The listing builds one solid part. Answer for the finished solid, in the listing's coordinates (mm). Round coordinates to 2 decimals unless told otherwise and drop trailing zeros. Loops run counter-clockwise (first coordinate to the right, second up) from the corner with the lowest first, then second, coordinate; pieces in that order, holes last. Notation, with made-up numbers: (60.5, -39.75) -> (86.5, -39.75) arc R14 ccw to (86.5, -17.75) -> close; hole circle Ø6 at (6.25, 65). An arc over 180 degrees is marked (long way). Use a Markdown table: item, result. Add a question column.
Q1. Section D-D on x = -4.75 is taken. Give the vertices of the cut face in (y, z).
Q2. Consider line 1 (X direction, y = 5.75, z = 0); line 2 (Z direction, x = -2.25, y = -1). Determine where each line is inside the solid, lowest interval first.
Q3. Section C-C on y = -1.5 is taken. Give the vertices of the cut face in (x, z), then the cut area to 3 significant figures.
Q4. Given pin 1 Ø8 at (y, z) = (-4.5, -6) entering from -X; pin 2 Ø5 at (x, y) = (3.5, -5) entering from -Z; pin 3 Ø5 at (y, z) = (4.5, -4) entering from -X, each flat-ended and moving along its own axis, determine where each tip first touches the part or whether it passes through.
Q5. Section A-A on x = 0 is taken. Give the vertices of the cut face in (y, z), then the cut area to 3 significant figures.
Q6. Section B-B on z = 1 is taken. Give the vertices of the cut face in (x, y).
from build123d import *

# Parameters (mm, degrees)
ESBO_O1_R                = 9.5
ESBO_O1_R_2              = 3.25
ESBO_O1_R_3              = 2.75
RESSALTO_EXTRUS_O1_DEPTH = 11


with BuildPart() as part:
    # Esboço1 → Ressalto-extrusão1 (new, symmetric)
    # profile 1 of 2: a face of its own
    with BuildSketch(Plane(origin=(0, 0, 0), x_dir=(1, 0, 0), z_dir=(0, 1, 0))):
        with Locations(Location((0, 0, 0), (0, 0, 270))):
            Circle(ESBO_O1_R)
        Circle(ESBO_O1_R_2, mode=Mode.SUBTRACT)
    # profile 2 of 2: a face of its own
    with BuildSketch(Plane(origin=(0, 0, 0), x_dir=(1, 0, 0), z_dir=(0, 1, 0))):
        Circle(ESBO_O1_R_2)
        with Locations(Location((0, 0, 0), (0, 0, 270))):
            Circle(ESBO_O1_R_3, mode=Mode.SUBTRACT)
    extrude(amount=RESSALTO_EXTRUS_O1_DEPTH, both=True)


solid = part.part
Checked values:
| question | item | result |
|---|---|---|
| 1 | outline | (-11, -8.23) -> (11, -8.23) -> (11, 8.23) -> (-11, 8.23) -> close |
| 2 | line 1 | x = -9.5 to -2.75, 2.75 to 9.5 |
| 2 | line 2 | z = -9.23 to -1.58, 1.58 to 9.23 |
| 3 | outline | circle Ø19 at (0, 0); hole circle Ø5.5 at (0, 0) |
| 3 | area | 260 mm2 |
| 4 | pin 1 | stops at x = -9.29 |
| 4 | pin 2 | stops at z = -9.45 |
| 4 | pin 3 | stops at x = -9.38 |
| 5 | outline | (-11, -9.5) -> (11, -9.5) -> (11, -2.75) -> (-11, -2.75) -> close; (-11, 2.75) -> (11, 2.75) -> (11, 9.5) -> (-11, 9.5) -> close |
| 5 | area | 297 mm2 |
| 6 | outline | (-9.45, -11) -> (-2.56, -11) -> (-2.56, 11) -> (-9.45, 11) -> close; (2.56, -11) -> (9.45, -11) -> (9.45, 11) -> (2.56, 11) -> close |
